Geometry check sheet. Reference: the model listing, model coordinates, mm. A direction names the side the tool comes from. Round coordinates to 2 decimals unless told otherwise and drop trailing zeros. Write each loop counter-clockwise with the first axis right and the second up, starting at its lowest first coordinate (ties: lowest second). Pieces come first, ordered by that corner, then holes. Notation, with made-up numbers: M 19,53.25 L 65,53.25 A21 ccw 65,57.25 Z; hole C 56.25,22 d2. An arc over 180 degrees is marked long. Answer in a Markdown table with one row per item. Add a question column.
Autodesk Inventor part; units mm, degrees
ref_plane "YZ Plane" through (0, 0, 0) normal (1, 0, 0) x (0, 1, 0)
ref_plane "XZ Plane" through (0, 0, 0) normal (0, 1, 0) x (-1, 0, 0)
ref_plane "XY Plane" through (0, 0, 0) normal (0, 0, 1) x (1, 0, 0)
sketch "Sketch1" plane through (0, 0, 0) normal (0, 1, 0) x (-1, 0, 0)
  line L0 (0, 0) -> (8, 0)
  line L1 (8, 0) -> (8, -25)
  line L2 (8, -25) -> (0, -25)
  line L3 (0, -25) -> (0, 0)
  dimension "d0" = 8
  dimension "d1" = 25
extrude "Extrusion1" add sketch "Sketch1" along normal blind 89
sketch "Sketch2" plane through (0, 0, 0) normal (1, 0, 0) x (0, 0, -1)
  line L0 (0, 89) -> (25, 89)
  line L1 (0, 89) -> (25, 89)
  line L2 (25, 89) -> (25, 64)
  line L3 (25, 64) -> (0, 64)
  line L4 (0, 64) -> (0, 89)
  line L5 (25, 0) -> (25, 89)
  line L6 (25, 0) -> (0, 0)
  line L7 (0, 0) -> (0, 25)
  line L8 (0, 25) -> (25, 25)
  line L9 (25, 25) -> (25, 0)
  dimension "d4" = 25
  dimension "d5" = 25
  dimension "d6" = 25
  dimension "d7" = 25
extrude "Extrusion2" add sketch "Sketch2" along normal blind 6
sketch "Sketch3" plane through (6, 0, 0) normal (1, 0, 0) x (0, 0, -1)
  line L0 (0, 0) -> (25, 0)
  line L1 (0, 0) -> (12.5, 0)
  line L2 (12.5, 0) -> (12.5, 12.5)
  circle A0 centre (12.5, 12.5) radius 2.5
  circle A1 centre (12.5, 76.5) radius 2.5
  line L3 (25, 89) -> (0, 89)
  line L4 (0, 89) -> (0, 64)
  dimension "d10" = 12.5
  dimension "d11" = 5
  dimension "d12" = 5
  dimension "d13" = 12.5
  dimension "d14" = 12.5
sketch "Sketch4" plane through (0, 25, -25) normal (1, 0, 0) x (0, 0, -1)
  circle A0 centre (-17, 19.5) radius 2.5
  line L0 (-25, -25) -> (0, -25)
  line L1 (-25, 0) -> (-25, 39)
  circle A1 centre (-8, 19.5) radius 2.5
  line L2 (0, 0) -> (0, 39)
  circle A2 centre (-12.5, 9.5) radius 2.5
  circle A3 centre (-12.5, 29.5) radius 2.5
  dimension "d15" = 5
  dimension "d16" = 44.5
  dimension "d17" = 8
  dimension "d18" = 5
  dimension "d19" = 8
  dimension "d20" = 44.5
  dimension "d21" = 5
  dimension "d22" = 5
  dimension "d23" = 10
  dimension "d24" = 4.5
  dimension "d25" = 10
  dimension "d26" = 4.5
extrude "Extrusion3" cut sketch "Sketch3" against normal up to next
extrude "Extrusion4" cut sketch "Sketch4" against normal up to next
sketch "Sketch5" plane through (0, 25, -25) normal (1, 0, 0) x (0, 0, -1)
  circle A0 centre (-12.5, 29.5) radius 2.5
  circle A1 centre (-12.5, 29.5) radius 4.5
  circle A2 centre (-17, 19.5) radius 2.5
  circle A3 centre (-17, 19.5) radius 4.5
  circle A4 centre (-8, 19.5) radius 2.5
  circle A5 centre (-8, 19.5) radius 4.5
  circle A6 centre (-12.5, 9.5) radius 2.5
  circle A7 centre (-12.5, 9.5) radius 4.5
  point P0 (-25, -25)
  dimension "d31" = 9
  dimension "d32" = 9
  dimension "d33" = 9
  dimension "d34" = 9
extrude "Extrusion5" cut sketch "Sketch5" against normal blind 4
properties part number "Back_Bracket_40mm" material "ABS Plastic"
Item 1: Access from +Z, -Z, +X, -X, +Y, -Y to the whole of each face (thin tool, end or side, straight path). Record for faces 1 (the flat face through (-4, 32.6, -14.4)), 2 (the cylindrical face through (-6, 54.6, -10)), 3 (the flat face through (3, 25, -12)).
Item 2: Section check D-D, the plane z = -23.5. Record the boundary of the cut face in (x, y), and give its area (3 significant figures).
Item 3: Section check A-A, the plane x = 3.25. Record the boundary of the cut face in (y, z), and give its area (3 significant figures).
Item 4: Gauge pin test, flat ends, axial feed: pin 1 Ø4.5 at (y, z) = (35, -11) entering from +X; pin 2 Ø14.5 at (y, z) = (54.5, -12.5) entering from +X. Record the tip position at first contact, or that the pin passes through.
Item 5: Section check B-B, the plane y = 76.5. Record the boundary of the cut face in (x, z), and give its area (3 significant figures).
Item 6: Scan lines: probe 1 along Y at (x, z) = (2.25, -12.5); probe 2 along Y at (x, z) = (-6.7, -12.5); probe 3 along X at (y, z) = (48.5, -7). Record each from-to range of solid material in increasing order. Write a range as from..to.
Item 7: Mould release check, pull along Z, two halves, no side actions. Record for faces 4 (the flat face through (-2, 44, 0)), 5 (the flat face through (-4, 52.6, -14.4)), 6 (the cylindrical face through (-0.9, 10.06, -11.96)), 7 (the flat face through (-1, 89, -12)): +Z half, -Z half, draft (parallel to the pull), parting line (faces both ways), or undercut.
Result sheet:
| question | item | result |
|---|---|---|
| 1 | face 1 | +X |
| 1 | face 2 | +X, -X |
| 1 | face 3 | +Z, -Z, +X |
| 2 | outline | M -8,0 L 6,0 L 6,25 L 0,25 L 0,64 L 6,64 L 6,89 L -8,89 Z |
| 2 | area | 1,010 mm^2 |
| 3 | outline | M 0,-25 L 25,-25 L 25,0 L 0,0 Z; M 64,-25 L 89,-25 L 89,0 L 64,0 Z; hole C 12.5,-12.5 d5; hole C 76.5,-12.5 d5 |
| 3 | area | 1,210 mm^2 |
| 4 | pin 1 | stops at x = -4 |
| 4 | pin 2 | stops at x = 0 |
| 5 | outline | M -8,-25 L 6,-25 L 6,-15 L -8,-15 Z; M -8,-10 L 6,-10 L 6,0 L -8,0 Z |
| 5 | area | 280 mm^2 |
| 6 | probe 1 | y = 0..10, 15..25, 64..74, 79..89 |
| 6 | probe 2 | y = 0..10, 15..32, 37..52, 57..74, 79..89 |
| 6 | probe 3 | x = -8..-4 |
| 7 | face 4 | +Z half |
| 7 | face 5 | undercut |
| 7 | face 6 | undercut |
| 7 | face 7 | draft |
